```python
from build123d import *

# Parameters (mm, degrees)
PAD019_DEPTH            = 6.2
SKETCH044_W             = 187.5
SKETCH044_H             = 187.5
PAD020_DEPTH            = 2.8
PAD021_DEPTH            = 8.5
BODY021_PLACEMENT_ANGLE = 90
PAD022_DEPTH            = 6.2
BODY023_PLACEMENT_ANGLE = 180
PAD028_DEPTH            = 2.3
PAD029_DEPTH            = 2.3
PAD030_DEPTH            = 2.3
PAD031_DEPTH            = 2.3
PAD032_DEPTH            = 2.3
PAD033_DEPTH            = 2.3
PAD034_DEPTH            = 8.5
SKETCH046_W             = 291
SKETCH046_H             = 291
PAD027_DEPTH            = 9.5
POCKET044_DEPTH         = 9.501


with BuildPart() as obj1:
    # Sketch043 → Pad019 (new body)
    with BuildSketch(Plane.XY):
        with BuildLine():
            Line((-51.25, 73.5), (51.25, 73.5))
            Line((51.25, 73.5), (51.25, -73.5))
            Line((51.25, -73.5), (14.832397, -73.5))
            ThreePointArc((-14.832397, -73.5), (0, -83.5), (14.832397, -73.5))
            Line((-14.832397, -73.5), (-51.25, -73.5))
            Line((-51.25, -73.5), (-51.25, 73.5))
        make_face()
    extrude(amount=PAD019_DEPTH)


with BuildPart() as obj1_1:
    # Body019 placement: moved
    add(obj1.part.moved(Location((92.65, 70.9, 3.3))))


with BuildPart() as obj2:
    # Sketch044 → Pad020 (new body)
    with BuildSketch(Plane.XY):
        Rectangle(SKETCH044_W, SKETCH044_H)
    extrude(amount=PAD020_DEPTH)


with BuildPart() as obj2_1:
    # Body020 placement: moved
    add(obj2.part.moved(Location((50.15, -50.15, 6.7))))


with BuildPart() as obj3:
    # Sketch045 → Pad021 (new body)
    with BuildSketch(Plane.XY):
        with BuildLine():
            Line((-58.8, 92.5), (58.8, 92.5))
            Line((58.8, 92.5), (58.8, -92.5))
            Line((58.8, -92.5), (17, -92.5))
            ThreePointArc((-17, -92.5), (0, -109.5), (17, -92.5))
            Line((-17, -92.5), (-58.8, -92.5))
            Line((-58.8, -92.5), (-58.8, 92.5))
        make_face()
    extrude(amount=PAD021_DEPTH)


with BuildPart() as obj3_1:
    # Body021 placement: moved
    add(obj3.part.moved(Location((50.15, -74, 1))).rotate(Axis((50.15, -74, 1), (0, 0, -1)), BODY021_PLACEMENT_ANGLE))


with BuildPart() as obj4:
    # Sketch047 → Pad022 (new body)
    with BuildSketch(Plane.XY):
        with BuildLine():
            Line((-51.25, 73.5), (-14.832397, 73.5))
            ThreePointArc((14.832397, 73.5), (0, 83.5), (-14.832397, 73.5))
            Line((14.832397, 73.5), (51.25, 73.5))
            Line((51.25, 73.5), (51.25, -73.5))
            Line((51.25, -73.5), (-51.25, -73.5))
            Line((-51.25, -73.5), (-51.25, 73.5))
        make_face()
    extrude(amount=PAD022_DEPTH)


with BuildPart() as obj4_1:
    # Body023 placement: moved
    add(obj4.part.moved(Location((-11.45, 70.9, 3.3))).rotate(Axis((-11.45, 70.9, 3.3), (0, 0, 1)), BODY023_PLACEMENT_ANGLE))


with BuildPart() as alliancetokens1:
    # Sketch054 → Pad028 (new body)
    with BuildSketch(Plane.XY):
        with BuildLine():
            ThreePointArc((8.5, -8.5), (24.025463, -17.7), (39.550926, -8.5))
            Line((51.25, -8.5), (39.550926, -8.5))
            Line((51.25, 8.5), (51.25, -8.5))
            Line((39.550926, 8.5), (51.25, 8.5))
            ThreePointArc((39.550926, 8.5), (24.025463, 17.7), (8.5, 8.5))
            Line((8.5, 8.5), (-8.5, 8.5))
            ThreePointArc((-8.5, 8.5), (-24.025463, 17.7), (-39.550926, 8.5))
            Line((-39.550926, 8.5), (-51.25, 8.5))
            Line((-51.25, 8.5), (-51.25, -8.5))
            Line((-51.25, -8.5), (-39.550926, -8.5))
            ThreePointArc((-39.550926, -8.5), (-24.025463, -17.7), (-8.5, -8.5))
            Line((8.5, -8.5), (-8.5, -8.5))
        make_face()
    extrude(amount=PAD028_DEPTH)


with BuildPart() as alliancetokens1_1:
    # Body028 placement: moved
    add(alliancetokens1.part.moved(Location((92.65, 106.5, 1))))


with BuildPart() as alliancetokens2:
    # Sketch055 → Pad029 (new body)
    with BuildSketch(Plane.XY):
        with BuildLine():
            ThreePointArc((8.5, -8.5), (24.025463, -17.7), (39.550926, -8.5))
            Line((51.25, -8.5), (39.550926, -8.5))
            Line((51.25, 8.5), (51.25, -8.5))
            Line((39.550926, 8.5), (51.25, 8.5))
            ThreePointArc((39.550926, 8.5), (24.025463, 17.7), (8.5, 8.5))
            Line((8.5, 8.5), (-8.5, 8.5))
            ThreePointArc((-8.5, 8.5), (-24.025463, 17.7), (-39.550926, 8.5))
            Line((-39.550926, 8.5), (-51.25, 8.5))
            Line((-51.25, 8.5), (-51.25, -8.5))
            Line((-51.25, -8.5), (-39.550926, -8.5))
            ThreePointArc((-39.550926, -8.5), (-24.025463, -17.7), (-8.5, -8.5))
            Line((8.5, -8.5), (-8.5, -8.5))
        make_face()
    extrude(amount=PAD029_DEPTH)


with BuildPart() as alliancetokens2_1:
    # Body029 placement: moved
    add(alliancetokens2.part.moved(Location((-11.45, 106.5, 1))))


with BuildPart() as obj5:
    # Sketch056 → Pad030 (new body)
    with BuildSketch(Plane.XY):
        Polygon((-39.5, 8.5), (-51.25, 8.5), (-51.25, -8.5), (-39.5, -8.5), (-39.5, -15.5), (-8.5, -15.5), (-8.5, -8.5), (8.5, -8.5), (8.5, -15.5), (39.5, -15.5), (39.5, -8.5), (51.25, -8.5), (51.25, 8.5), (39.5, 8.5), (39.5, 15.5), (8.5, 15.5), (8.5, 8.5), (-8.5, 8.5), (-8.5, 15.5), (-39.5, 15.5), align=None)
    extrude(amount=PAD030_DEPTH)


with BuildPart() as obj5_1:
    # Body030 placement: moved
    add(obj5.part.moved(Location((92.65, 66.7, 1))))


with BuildPart() as obj6:
    # Sketch057 → Pad031 (new body)
    with BuildSketch(Plane.XY):
        Polygon((-39.5, 8.5), (-51.25, 8.5), (-51.25, -8.5), (-39.5, -8.5), (-39.5, -15.5), (-8.5, -15.5), (-8.5, -8.5), (8.5, -8.5), (8.5, -15.5), (39.5, -15.5), (39.5, -8.5), (51.25, -8.5), (51.25, 8.5), (39.5, 8.5), (39.5, 15.5), (8.5, 15.5), (8.5, 8.5), (-8.5, 8.5), (-8.5, 15.5), (-39.5, 15.5), align=None)
    extrude(amount=PAD031_DEPTH)


with BuildPart() as obj6_1:
    # Body031 placement: moved
    add(obj6.part.moved(Location((-11.45, 66.7, 1))))


with BuildPart() as obj7:
    # Sketch058 → Pad032 (new body)
    with BuildSketch(Plane.XY):
        with BuildLine():
            Line((-19.965971, 8.5), (-36.965971, 8.5))
            Line((-36.965971, 8.5), (-36.965971, -8.5))
            Line((-36.965971, -8.5), (-19.965971, -8.5))
            ThreePointArc((-19.965971, -8.5), (0, -21.7), (19.965971, -8.5))
            Line((36.965971, -8.5), (19.965971, -8.5))
            Line((36.965971, 8.5), (36.965971, -8.5))
            Line((19.965971, 8.5), (36.965971, 8.5))
            ThreePointArc((19.965971, 8.5), (0, 21.7), (-19.965971, 8.5))
        make_face()
    extrude(amount=PAD032_DEPTH)


with BuildPart() as obj7_1:
    # Body032 placement: moved
    add(obj7.part.moved(Location((92.65, 22.7, 1))))


with BuildPart() as obj8:
    # Sketch059 → Pad033 (new body)
    with BuildSketch(Plane.XY):
        Polygon((-28.5, 8.5), (-38.5, 8.5), (-38.5, -8.5), (-28.5, -8.5), (-28.5, -15), (28.5, -15), (28.5, -8.5), (38.5, -8.5), (38.5, 8.5), (28.5, 8.5), (28.5, 15), (-28.5, 15), align=None)
    extrude(amount=PAD033_DEPTH)


with BuildPart() as obj8_1:
    # Body033 placement: moved
    add(obj8.part.moved(Location((-11.45, 22.7, 1))))


with BuildPart() as obj9:
    # Sketch060 → Pad034 (new body)
    with BuildSketch(Plane.XY):
        with BuildLine():
            Line((-33.75, 143.9), (33.75, 143.9))
            Line((33.75, 143.9), (33.75, 51.4))
            Line((33.75, 51.4), (10, 51.4))
            ThreePointArc((10, 51.4), (7.425, 48.825), (10, 46.25))
            Line((10, 46.25), (33.75, 46.25))
            Line((33.75, 46.25), (33.75, -46.25))
            Line((33.75, -46.25), (10, -46.25))
            ThreePointArc((10, -46.25), (7.425, -48.825), (10, -51.4))
            Line((10, -51.4), (33.75, -51.4))
            Line((33.75, -51.4), (33.75, -143.9))
            Line((33.75, -143.9), (-33.75, -143.9))
            Line((-33.75, -143.9), (-33.75, -113.555974))
            ThreePointArc((-33.75, -81.744026), (-44.75, -97.65), (-33.75, -113.555974))
            Line((-33.75, -81.744026), (-33.75, -51.4))
            Line((-33.75, -51.4), (-10, -51.4))
            ThreePointArc((-10, -51.4), (-7.425, -48.825), (-10, -46.25))
            Line((-10, -46.25), (-33.75, -46.25))
            Line((-33.75, -46.25), (-33.75, -15.905974))
            ThreePointArc((-33.75, 15.905974), (-44.75, 0), (-33.75, -15.905974))
            Line((-33.75, 15.905974), (-33.75, 46.25))
            Line((-33.75, 46.25), (-10, 46.25))
            ThreePointArc((-10, 46.25), (-7.425, 48.825), (-10, 51.4))
            Line((-10, 51.4), (-33.75, 51.4))
            Line((-33.75, 51.4), (-33.75, 81.744026))
            ThreePointArc((-33.75, 113.555974), (-44.75, 97.65), (-33.75, 81.744026))
            Line((-33.75, 113.555974), (-33.75, 143.9))
        make_face()
    extrude(amount=PAD034_DEPTH)


with BuildPart() as obj9_1:
    # Body034 placement: moved
    add(obj9.part.moved(Location((-99.15, 0, 1))))


with BuildPart() as topinsert:
    # Sketch046 → Pad027 (new body)
    with BuildSketch(Plane.XY):
        Rectangle(SKETCH046_W, SKETCH046_H)
    extrude(amount=PAD027_DEPTH)

    # Boolean: cut obj1, obj2, obj3, obj4, AllianceTokens1, AllianceTokens2, obj5, obj6, obj7, obj8, obj9
    add(obj1_1.part, mode=Mode.SUBTRACT)
    add(obj2_1.part, mode=Mode.SUBTRACT)
    add(obj3_1.part, mode=Mode.SUBTRACT)
    add(obj4_1.part, mode=Mode.SUBTRACT)
    add(alliancetokens1_1.part, mode=Mode.SUBTRACT)
    add(alliancetokens2_1.part, mode=Mode.SUBTRACT)
    add(obj5_1.part, mode=Mode.SUBTRACT)
    add(obj6_1.part, mode=Mode.SUBTRACT)
    add(obj7_1.part, mode=Mode.SUBTRACT)
    add(obj8_1.part, mode=Mode.SUBTRACT)
    add(obj9_1.part, mode=Mode.SUBTRACT)

    # Sketch123 → Pocket044 (cut, through all)
    with BuildSketch(Plane.XY):
        Polygon((-145.5, 145.5), (-145.5, 0), (-145.5, -145.5), (0, -145.5), (0, -87.75), (-10, -97.75), (-10, -47.75), (0, -57.75), (0, 0), (57.75, 0), (47.75, -10), (97.75, -10), (87.75, 0), (145.5, 0), (145.5, 145.5), (0, 145.5), align=None)
    extrude(amount=POCKET044_DEPTH, mode=Mode.SUBTRACT)


solid = topinsert.part
```
CAD build for the part. Positions are in the model's coordinates, mm. A direction names the side the tool comes from. Give positions to 0.01 mm unless a question says otherwise; leave off trailing zeros. Loops run counter-clockwise (first coordinate to the right, second up) from the corner with the lowest first, then second, coordinate; pieces in that order, holes last. Notation, with made-up numbers: M 1.5,-16 L 42.5,-16 A20 ccw 42.5,-1 Z; hole C 37.25,-26.75 d4. An arc over 180 degrees is marked long. Use one line per item in the form item = value.
Item 1: Slice it at B-B (z = 4.75). List the corners of the cut face in (x, y), plus the area to 3 significant figures.
Determined:
outline = M 0,-145.5 L 145.5,-145.5 L 145.5,0 L 143.9,0 L 143.9,-2.6 L 107.48,-2.6 A16 cw 83.91,-10 L 47.75,-10 L 55.15,-2.6 L 41.4,-2.6 L 41.4,0 L 39.8,0 L 39.8,-2.6 L 3.38,-2.6 A16 cw 0,-7.78 L 0,-15.2 L 142.65,-15.2 L 142.65,-132.8 L 0,-132.8 Z
area = 3,590 mm2
Item 2: Two-plate mould, pull along X, no slides. Class faces 1 (the face through (-4.93, -92.68, 0.49)), 2 (the face through (92.82, -5.07, 1.63)), 3 (the face through (142.65, -73, 4)), 4 (the face through (67, -75, 1)): pulls with the +X half, pulls with the -X half, needs draft (parallel to the pull), parting line crosses it, or undercut.
Determined:
face_1 = undercut
face_2 = undercut
face_3 = pulls with the -X half
face_4 = needs draft
Item 3: Flat gauge pins, fed straight in: pin 1 (0.8 mm diameter, centred on x = 69, z = 8, fed in from +Y); pin 2 (14 mm diameter, centred on x = 124.5, y = -9, fed in from +Z); pin 3 (3.5 mm diameter, centred on x = 82, z = 2.5, fed in from +Y). Where does each tip first touch, or does it go through?
Determined:
pin_1 = -143.9
pin_2 = 6.7
pin_3 = -10
Item 4: Which spindle directions (+Z, -Z, +X, -X, +Y, -Y) get a long thin tool onto all of the face, cutting with end or side? Do faces 5 (the face through (110, -2, 3.3)), 6 (the face through (70, -15.2, 4)), 7 (the face through (20, -1, 3.3)). Say none if no direction does.
Determined:
face_5 = +Z, +Y
face_6 = +Z, -X
face_7 = +Z, -X, +Y
Item 5: Slice it at D-D (x = 80.5). List the corners of the cut face in (y, z), plus the area to 3 significant figures.
Determined:
outline = M -145.5,0 L -10,0 L -10,6.7 L -15.2,6.7 L -15.2,1 L -132.8,1 L -132.8,6.7 L -143.9,6.7 L -143.9,9.5 L -145.5,9.5 Z
area = 242 mm2
Item 6: Slice it at C-C (y = -40). List the corners of the cut face in (x, z), plus the area to 3 significant figures.
Determined:
outline = M 0,0 L 145.5,0 L 145.5,9.5 L 143.9,9.5 L 143.9,6.7 L 142.65,6.7 L 142.65,1 L 0,1 Z
area = 166 mm2
Item 7: Slice it at A-A (x = 114). List the corners of the cut face in (y, z), plus the area to 3 significant figures.
Determined:
outline = M -145.5,0 L 0,0 L 0,3.3 L -2.6,3.3 L -2.6,6.7 L -15.2,6.7 L -15.2,1 L -132.8,1 L -132.8,6.7 L -143.9,6.7 L -143.9,9.5 L -145.5,9.5 Z
area = 300 mm2
Item 8: Drill centre lines: probe 1 along Y at (x, z) = (19, 6.5); probe 2 along Y at (x, z) = (102.5, 2.25); probe 3 along X at (y, z) = (-7, 8.25). Where is each one in solid material? Low to high. Write a range as from..to.
Determined:
probe_1 = -145.5..-132.8, -15.2..-2.6
probe_2 = -145.5..-132.8, -15.2..0
probe_3 = 143.9..145.5
